The model under review builds one solid part; all positions refer to its coordinate system, in mm. A direction names the side the tool comes from. Round coordinates to 2 decimals unless told otherwise and drop trailing zeros. Loops run counter-clockwise (first coordinate to the right, second up) from the corner with the lowest first, then second, coordinate; pieces in that order, holes last. Notation, with made-up numbers: M -26,13 L 15,13 A37 ccw 15,52 Z; hole C 67.5,51.5 d11. An arc over 180 degrees is marked long. Use a Markdown table: item, result. Add a question column.
Autodesk Inventor part; units mm, degrees
ref_plane "YZ Plane" through (0, 0, 0) normal (1, 0, 0) x (0, 1, 0)
ref_plane "XZ Plane" through (0, 0, 0) normal (0, 1, 0) x (-1, 0, 0)
ref_plane "XY Plane" through (0, 0, 0) normal (0, 0, 1) x (1, 0, 0)
sketch "Sketch1" plane through (0, 0, 0) normal (0, 1, 0) x (-1, 0, 0)
  line L0 (0, 0) -> (25, 0)
  line L1 (25, 0) -> (25, -76)
  line L2 (25, -76) -> (0, -76)
  line L3 (0, -76) -> (0, 0)
  dimension "d0" = 76
  dimension "d1" = 25
extrude "Extrusion1" add sketch "Sketch1" along normal blind 2.5
ref_plane "Work Plane2" through (0, 5.5, 0) normal (0, 1, 0) x (1, 0, 0)
sketch "Sketch3" plane through (0, 5.5, 0) normal (0, 1, 0) x (1, 0, 0)
  line L0 (0, 0) -> (-25, 0) construction
  line L1 (-12.5, 0) -> (-12.5, 76) construction
  line L2 (-25, 76) -> (0, 76) construction
  line L3 (-25, 71) -> (-25, 5) construction
  line L4 (-25, 38) -> (-0.4405, 38) construction
  line L5 (-20, 28.5) -> (-5, 28.5)
  line L6 (-3, 30.5) -> (-3, 45.5)
  line L7 (-5, 47.5) -> (-20, 47.5)
  line L8 (-22, 45.5) -> (-22, 30.5)
  line L9 (-22, 28.5) -> (-3, 47.5) construction
  line L10 (-3, 28.5) -> (-22, 47.5) construction
  arc A0 (-20, 47.5) -> (-22, 45.5) centre (-20, 45.5) ccw
  arc A1 (-3, 45.5) -> (-5, 47.5) centre (-5, 45.5) ccw
  arc A2 (-5, 28.5) -> (-3, 30.5) centre (-5, 30.5) ccw
  arc A3 (-22, 30.5) -> (-20, 28.5) centre (-20, 30.5) ccw
  point P0 (-12.5, 38)
  dimension "d8" = 19
  dimension "d9" = 2
  dimension "d10" = 2
  dimension "d11" = 2
  dimension "d12" = 2
extrude "Extrusion3" cut sketch "Sketch3" against normal blind 6
sketch "Sketch4" plane through (0, 0, 0) normal (0, -1, 0) x (1, 0, 0)
  line L0 (0, -76) -> (0, 0) construction
  line L1 (0, -38) -> (-25, -38) construction
  line L2 (-25, -71) -> (-25, -5) construction
  line L3 (0, 0) -> (-25, 0) construction
  line L4 (-12.5, 0) -> (-12.5, -76) construction
  line L5 (-25, -76) -> (0, -76) construction
  line L6 (-19.875, -49.375) -> (-5.125, -49.375)
  line L7 (-1.125, -49.375) -> (-1.125, -26.625)
  line L8 (-5.125, -26.625) -> (-19.875, -26.625)
  line L9 (-23.875, -26.625) -> (-23.875, -49.375)
  line L10 (-23.875, -49.375) -> (-1.125, -26.625) construction
  line L11 (-1.125, -49.375) -> (-23.875, -26.625) construction
  arc A0 (-1.125, -26.625) -> (-5.125, -26.625) centre (-3.125, -26.625) ccw
  arc A1 (-19.875, -26.625) -> (-23.875, -26.625) centre (-21.875, -26.625) ccw
  arc A2 (-23.875, -49.375) -> (-19.875, -49.375) centre (-21.875, -49.375) ccw
  arc A3 (-5.125, -49.375) -> (-1.125, -49.375) centre (-3.125, -49.375) ccw
  point P0 (-12.5, -38)
  dimension "d15" = 22.75
  dimension "d16" = 4
  dimension "d17" = 22.75
extrude "Extrusion4" cut sketch "Sketch4" against normal blind 0.5
sketch "Sketch5" plane through (0, 0, 0) normal (0, -1, 0) x (1, 0, 0)
  circle A0 centre (-12.5, -19.3349) radius 2.5305
  circle A1 centre (-12.5, -56) radius 2.6164
  line L0 (0, -76) -> (0, 0)
  line L1 (-25, -76) -> (0, -76)
  dimension "d20" = 12.5
  dimension "d21" = 20
properties part number "scope coverslip holder lowpro"
(1) For faces 5 (the face through (-22, 2, -38)), 6 (the face through (-21.831, 0.246, -24.625)), 7 (the face through (-12, 0, -54)), list the 3-axis set-ups (+Z, -Z, +X, -X, +Y, -Y) from which the entire face can be reached by the end or side of a thin tool; tool diameter is ignored.
(2) Consider section D-D, the plane x = -23. Give the boundary of the cut face in (y, z), then the cut area to 3 significant figures.
(3) To check wall thickness, follow probe 1 along Z at (x, y) = (-3, 0.3); probe 2 along Z at (x, y) = (-12.25, 1.4); probe 3 along X at (y, z) = (0.35, -42) (3 decimals). State the ranges of each line that lie inside material, in increasing order.
(4) Draft analysis for pull direction X (two halves, no side actions). For faces 1 (the face through (-3, 2, -38)), 2 (the face through (-3.6, 1.51, -29.07)), 3 (the face through (0, 1, -39)), 4 (the face through (-13, 1, -76)), state which applies: released by +X, released by -X, zero draft, split by the parting line, or undercut.
(5) Consider section C-C, the plane z = -39. Give the boundary of the cut face in (x, y) (3 decimals).
(6) Consider section A-A, the plane x = -9. Give the boundary of the cut face in (y, z) (3 decimals).
(7) Consider section B-B, the plane y = 2. Give the boundary of the cut face in (x, z).
(8) Insertion check: pin 1 Ø11.5 at (x, z) = (-15.5, -32.5) entering from -Y. The pin has a flat end and moves straight along its axis. Give the tip position at first contact, or say it passes through.
Found:
| question | item | result |
|---|---|---|
| 1 | face 5 | +Y, -Y |
| 1 | face 6 | -Y |
| 1 | face 7 | +Z, -Z, +X, -X, -Y |
| 2 | outline | M 0,-76 L 2.5,-76 L 2.5,0 L 0,0 L 0,-24.97 L 0.5,-24.97 L 0.5,-51.03 L 0,-51.03 Z |
| 2 | area | 177 mm^2 |
| 3 | probe 1 | z = -76 to -51.37, -24.63 to 0 |
| 3 | probe 2 | z = -76 to -47.5, -28.5 to 0 |
| 3 | probe 3 | x = -25 to -23.875, -1.125 to 0 |
| 4 | face 1 | undercut |
| 4 | face 2 | undercut |
| 4 | face 3 | released by +X |
| 4 | face 4 | zero draft |
| 5 | outline | M -25,0 L -23.875,0 L -23.875,0.5 L -22,0.5 L -22,2.5 L -25,2.5 Z; M -3,0.5 L -1.125,0.5 L -1.125,0 L 0,0 L 0,2.5 L -3,2.5 Z |
| 6 | outline | M 0,-76 L 2.5,-76 L 2.5,-47.5 L 0.5,-47.5 L 0.5,-49.375 L 0,-49.375 Z; M 0,-26.625 L 0.5,-26.625 L 0.5,-28.5 L 2.5,-28.5 L 2.5,0 L 0,0 Z |
| 7 | outline | M -25,-76 L 0,-76 L 0,0 L -25,0 Z; hole M -22,-45.5 A2 ccw -20,-47.5 L -5,-47.5 A2 ccw -3,-45.5 L -3,-30.5 A2 ccw -5,-28.5 L -20,-28.5 A2 ccw -22,-30.5 Z |
| 8 | pin 1 | stops at y = 0.5 |
